```python
from build123d import *

# Parameters (mm, degrees)
TIBIA_RAW_DEPTH                 = 7.5
ARRONDISSEMENT_PATTE_DEPTH      = 141.261849538
ARRONDISSEMENT_PATTE_DEPTH_BACK = 141.261849538
SKETCH10_W                      = 25.4
SKETCH10_H                      = 35
BOSS_EXTRUDE3_DEPTH             = 5
SKETCH11_R                      = 15
CUT_EXTRUDE3_DEPTH              = 5
F_3_0MM_DOWEL_HOLE2_D           = 3
F_3_0MM_DOWEL_HOLE2_CSINK_D     = 3.05
F_3_0MM_DOWEL_HOLE2_CSINK_ANGLE = 90
RIB2_REACH                      = 154.986
SKETCH14_WALL_W                 = 319.8505485
SKETCH14_WALL_H                 = 5


with BuildPart() as part:
    # Sketch1 → tibia_raw (new, symmetric)
    with BuildSketch(Plane.XY):
        Polygon((-8.044335554, 0), (-8.044335554, 25), (-47.248988291, 92.904450435), (-64.926657821, 110.582119965), (-51.405330856, 124.10344693), (16.455664446, 6.564755215), align=None)
    extrude(amount=TIBIA_RAW_DEPTH, both=True)

    # Sketch4 → arrondissement_patte (cut, two sides: drawn at the far end of the back side and taken through both)
    with BuildSketch(Plane.XY.offset(-ARRONDISSEMENT_PATTE_DEPTH_BACK)):
        with BuildLine():
            ThreePointArc((4.205663462, 3.282377343), (-1.866483675, 2.074552283), (-8.044335554, 1.669634512))
            Line((-8.044335554, 1.669634512), (-8.044335554, 0))
            Line((-8.044335554, 0), (4.205663462, 3.282377343))
        make_face()
        with BuildLine():
            ThreePointArc((15.620847191, 8.010701117), (10.068210696, 5.272443864), (4.205663462, 3.282377343))
            Line((4.205663462, 3.282377343), (16.455664446, 6.564755215))
            Line((16.455664446, 6.564755215), (15.620847191, 8.010701117))
        make_face()
    extrude(amount=ARRONDISSEMENT_PATTE_DEPTH + ARRONDISSEMENT_PATTE_DEPTH_BACK, mode=Mode.SUBTRACT)

    # Sketch10 → Boss-Extrude3 (add)
    with BuildSketch(Plane(origin=(-87.754388893, 87.754388893, 0), x_dir=(0, 0, 1), z_dir=(-0.7071067811865487, 0.7071067811865465, 0))):
        with Locations((0, 41.844308868)):
            Rectangle(SKETCH10_W, SKETCH10_H)
    extrude(amount=BOSS_EXTRUDE3_DEPTH)

    # Sketch11 → Cut-Extrude3 (cut, symmetric)
    with BuildSketch(Plane.XY):
        with Locations((-47.559392621, 131.484919071)):
            Circle(SKETCH11_R)
    extrude(amount=CUT_EXTRUDE3_DEPTH, both=True, mode=Mode.SUBTRACT)

    # Ø3.0mm Dowel Hole2 (through all)
    with Locations(Plane(origin=(-91.289922799, 91.289922799, 0), x_dir=(0, 0, 1), z_dir=(-0.7071067811865488, 0.7071067811865464, 0))):
        with Locations((-9.525, 55.314308868), (9.525, 55.314308868), (9.525, 28.374308868), (-9.525, 28.374308868)):
            CounterSinkHole(F_3_0MM_DOWEL_HOLE2_D / 2, F_3_0MM_DOWEL_HOLE2_CSINK_D / 2, counter_sink_angle=F_3_0MM_DOWEL_HOLE2_CSINK_ANGLE)

    # Sketch14 wall → Rib2 (add, up to next)
    with BuildSketch(Plane(origin=(-63.389537203, 104.845507721, 0), x_dir=(0.965925826292, -0.258819045091, 0), z_dir=(0.258819045091, 0.965925826292, 0)), mode=Mode.PRIVATE) as rib2_sk1:
        Rectangle(SKETCH14_WALL_W, SKETCH14_WALL_H)
    rib2_tool1 = extrude(rib2_sk1.sketch, amount=RIB2_REACH, mode=Mode.PRIVATE) - part.part
    add(rib2_tool1.solids().sort_by_distance((-63.389537203, 104.845507721, 0))[0])


solid = part.part
```
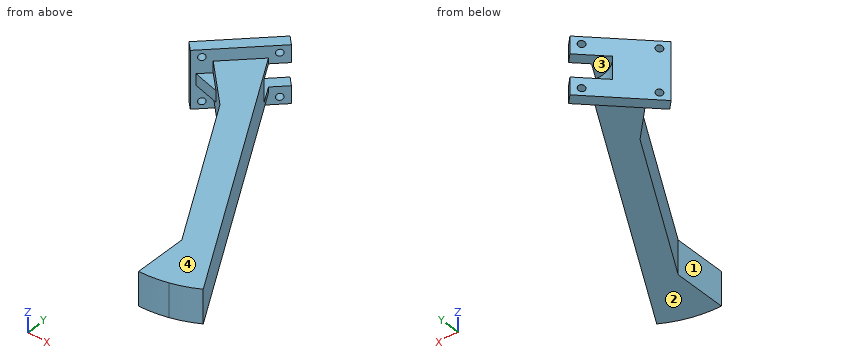
Could you check a few things on this model? Use its own coordinates, in mm. Face numbers are marked on the shaded views. A direction names the side the tool comes from. Coordinates: 2 decimals unless noted, no trailing zeros. Write each loop counter-clockwise with the first axis right and the second up, starting at its lowest first coordinate (ties: lowest second). Pieces come first, ordered by that corner, then holes. Notation, with made-up numbers: (6, -35.75) -> (41, -35.75) arc R6 cw to (41, -28.75) -> close; hole circle Ø4 at (62, 41.25). An arc over 180 degrees is marked (long way). Return JSON: item names as keys, results as strings.
(1) Imagine slicing it at A-A, the plane z = -0.75. Please give me the cut outline in (x, y).
Numbers:
{"outline": "(-74.08, 108.5) -> (-70.54, 104.97) -> (-69.13, 106.38) -> (-57.65, 103.31) -> (-47.25, 92.9) -> (-8.04, 25) -> (-8.04, 1.67) arc R47.33 ccw to (15.62, 8.01) -> (-47.01, 116.49) arc R15 cw to (-59.79, 122.79) -> close"}
(2) Imagine slicing it at C-C, the plane y = 102. Please give me the cut outline in (x, z).
Numbers:
{"outline": "(-56.34, -7.5) -> (-38.64, -7.5) -> (-38.64, 7.5) -> (-56.34, 7.5) -> close"}
(3) Which directions (+Z, -Z, +X, -X, +Y, -Y) give clear straight access to the entire face, cutting with the end or side of a thin tool? Please do the marked faces 1, 2, 3 and 4.
Numbers:
{"face 1": "+Z, -Z, -X, -Y", "face 2": "-Z, +X, -Y", "face 3": "+X, +Y", "face 4": "+Z, +X, -Y"}
(4) I need wall thicknesses on L1, parallel to Y at x = -48, z = 6.25; L2, parallel to Z at x = -9, y = 27; L3, parallel to X at y = 54, z = -3. Which ranges of each line are inside material? Lowest first, please.
Numbers:
{"L1": "y = 93.66 to 118.21, 127.51 to 131.93", "L2": "z = -7.5 to 7.5", "L3": "x = -24.79 to -10.93"}
(5) I'm going to push flat-ended pins straight in: pin 1 (5 mm diameter, centred on x = -54.5, z = -6, fed in from -Y); pin 2 (4.5 mm diameter, centred on y = 14.5, z = 2, fed in from -X); pin 3 (1 mm diameter, centred on x = -2, z = 9.5, fed in from -Y); pin 4 (1 mm diameter, centred on y = 31, z = -5.5, fed in from +X). Where does each tip first touch, or does it pass through?
Numbers:
{"pin 1": "stops at y = 97.66", "pin 2": "stops at x = -8.04", "pin 3": "passes through", "pin 4": "stops at x = 2.64"}
(6) Imagine slicing it at B-B, the plane x = -63.5. Please give me the cut outline in (y, z).
Numbers:
{"outline": "(104.88, -2.5) -> (109.16, -2.5) -> (109.16, -7.5) -> (112.01, -7.5) -> (112.01, -12.7) -> (119.08, -12.7) -> (119.08, 12.7) -> (112.01, 12.7) -> (112.01, 7.5) -> (109.16, 7.5) -> (109.16, 2.5) -> (104.88, 2.5) -> close"}
(7) Imagine slicing it at D-D, the plane x = -42. Please give me the cut outline in (y, z).
Numbers:
{"outline": "(83.81, -7.5) -> (107.81, -7.5) -> (107.81, 7.5) -> (83.81, 7.5) -> close"}
